from build123d import *

# Parameters (mm, degrees)
SKETCH1_R               = 4.75
BOSS_EXTRUDE1_DEPTH     = 9.5
SKETCH2_W               = 19
SKETCH2_H               = 9.5
CUT_EXTRUDE1_DEPTH      = 11
CUT_EXTRUDE1_DEPTH_BACK = 11
CHAMFER1_SIZE           = 8
CHAMFER1_SIZE2          = 1.895543273
CHAMFER2_SIZE           = 8
CHAMFER2_SIZE2          = 1.846945529
SKETCH5_R               = 1.5
CUT_EXTRUDE2_DEPTH      = 10.5000001
CUT_EXTRUDE2_DEPTH_BACK = 10.5000001


with BuildPart() as part:
    # Sketch1 → Boss-Extrude1 (new body, symmetric)
    with BuildSketch(Plane.XY):
        with BuildLine():
            Line((0, 10), (-22, 10))
            Line((-22, 10), (-22, 5))
            Line((-22, 5), (-9.9979998, 0.2))
            ThreePointArc((-9.9979998, 0.2), (-6.49865122, -7.600495531), (1.750767609, -9.845547866))
            Line((1.750767609, -9.845547866), (29, -5))
            Line((29, -5), (29, 0))
            Line((29, 0), (10, 0))
            ThreePointArc((10, 0), (7.071067812, 7.071067812), (0, 10))
        make_face()
        Circle(SKETCH1_R, mode=Mode.SUBTRACT)
    extrude(amount=BOSS_EXTRUDE1_DEPTH, both=True)

    # Sketch2 → Cut-Extrude1 (cut, two sides)
    with BuildSketch(Plane(origin=(0, 0, 0), x_dir=(1, 0, 0), z_dir=(0, 1, 0))) as cut_extrude1_sk:
        with Locations((-22, 0)):
            Rectangle(SKETCH2_W, SKETCH2_H)
        with Locations((29, 0)):
            Rectangle(SKETCH2_W, SKETCH2_H)
        with BuildLine():
            Line((-6, 5), (4, 5))
            ThreePointArc((4, 5), (9, 0), (4, -5))
            Line((4, -5), (-6, -5))
            ThreePointArc((-6, -5), (-11, 0), (-6, 5))
        make_face()
    extrude(amount=CUT_EXTRUDE1_DEPTH, mode=Mode.SUBTRACT)
    extrude(cut_extrude1_sk.sketch, amount=-CUT_EXTRUDE1_DEPTH_BACK, mode=Mode.SUBTRACT)

    # Chamfer1
    chamfer1_edges = [part.edges().sort_by_distance(p)[0] for p in [
        (-22, 7.5, 9.5),
        (29, -2.5, 9.5),
    ]]
    chamfer1_side = [part.faces().sort_by_distance(p)[0] for p in [
        (6.683704933, 6.683704933, 9.5),
    ]]
    chamfer(chamfer1_edges, length=CHAMFER1_SIZE, length2=CHAMFER1_SIZE2, reference=chamfer1_side[0])

    # Chamfer2
    chamfer2_edges = [part.edges().sort_by_distance(p)[0] for p in [
        (-22, 7.5, -9.5),
        (29, -2.5, -9.5),
    ]]
    chamfer2_side = [part.faces().sort_by_distance(p)[0] for p in [
        (6.683704933, 6.683704933, -9.5),
    ]]
    chamfer(chamfer2_edges, length=CHAMFER2_SIZE, length2=CHAMFER2_SIZE2, reference=chamfer2_side[0])

    # Sketch5 → Cut-Extrude2 (cut, two sides)
    with BuildSketch(Plane.XY) as cut_extrude2_sk:
        with Locations((-19.684598733, 7.5)):
            Circle(SKETCH5_R)
        with Locations((26.44619669, -2.5)):
            Circle(SKETCH5_R)
    extrude(amount=CUT_EXTRUDE2_DEPTH, mode=Mode.SUBTRACT)
    extrude(cut_extrude2_sk.sketch, amount=-CUT_EXTRUDE2_DEPTH_BACK, mode=Mode.SUBTRACT)


solid = part.part
Check sheet for the modelled part. Datum: model origin and axes. Units: mm. A direction names the side the tool comes from. Round coordinates to 2 decimals unless told otherwise and drop trailing zeros. Loops run counter-clockwise (first coordinate to the right, second up) from the corner with the lowest first, then second, coordinate; pieces in that order, holes last.
1. Gauge pin test, flat ends, axial feed: pin 1 Ø1 at (y, z) = (2.5, 3.5) entering from -X; pin 2 Ø8 at (y, z) = (-5.5, -2) entering from -X; pin 3 Ø5.5 at (x, y) = (26.5, -4.5) entering from +Z; pin 4 Ø2.5 at (x, y) = (-19.68, 7.5) entering from -Z. Record the tip position at first contact, or that the pin passes through.
2. Sectioned sample at D-D on y = 3.5. Record the boundary of the cut face in (x, z), and give its area (3 significant figures).
3. Sectioned sample at A-A on z = -0.5. Record the boundary of the cut face in (x, y).
4. Set-up check for faces 1 (the flat face through (-16, 7, 4.75)), 2 (the flat face through (18, 0, 0)), 3 (the flat face through (23, -3, 4.75)): record each of +Z, -Z, +X, -X, +Y, -Y from which the full face is reachable in a straight line by a thin tool's end or side.
5. Sectioned sample at C-C on x = 6. Record the boundary of the cut face in (y, z).
6. Mould release check, pull along Y, two halves, no side actions. Record for faces 4 (the flat face through (24.17, -3.26, -8.77)), 5 (the cylindrical face through (9.109, 4.126, 2.244)), 6 (the cylindrical face through (24.948, -2.434, 6.647)): released by +Y, released by -Y, zero draft, split by the parting line, or undercut.
7. Scan lines: probe 1 along Z at (x, y) = (-0.5, 8.5); probe 2 along X at (y, z) = (-2.5, 7.45); probe 3 along Z at (x, y) = (-13, 3). Record each from-to range of solid material in increasing order.
8. Sectioned sample at B-B on y = 7.5. Record the boundary of the cut face in (x, z), and give its area (3 significant figures).
Recorded:
1. pin 1: stops at x = -12.5
1. pin 2: stops at x = -9.86
1. pin 3: stops at z = 8.85
1. pin 4: passes through
2. outline: (-18.25, -8.52) - (-14, -9.5) - (-3.21, -9.5) - (-3.21, -5) - (-6, -5) arc R5 cw to (-6, 5) - (-3.21, 5) - (-3.21, 9.5) - (-14, 9.5) - (-18.25, 8.49) - (-18.25, 4.75) - (-12.5, 4.75) - (-12.5, -4.75) - (-18.25, -4.75) - close; (3.21, -9.5) - (9.37, -9.5) - (9.37, 9.5) - (3.21, 9.5) - (3.21, 5) - (4, 5) arc R5 cw to (4, -5) - (3.21, -5) - close
2. area: 230 mm2
3. outline: (-12.5, 1.2) - (-10.97, 0.59) - (-10.97, 10) - (-12.5, 10) - close; (8.97, -8.56) - (19.5, -6.69) - (19.5, 0) - (10, 0) arc R10 ccw to (8.97, 4.41) - close
4. face 1: -X, +Y, -Y
4. face 2: +Z, -Z, +X, +Y
4. face 3: +X, +Y, -Y
5. outline: (-9.09, -9.5) - (8, -9.5) - (8, -4.58) - (-9.09, -4.58) - close; (-9.09, 4.58) - (8, 4.58) - (8, 9.5) - (-9.09, 9.5) - close
6. face 4: zero draft
6. face 5: released by +Y
6. face 6: undercut
7. probe 1: z = -9.5 to -5, 5 to 9.5
7. probe 2: x = -9.68 to -4.04, 4.04 to 24.95, 27.95 to 29
7. probe 3: z = -9.5 to -4.75, 4.75 to 9.5
8. outline: (-22, -7.65) - (-21.18, -7.84) - (-21.18, -4.75) - (-22, -4.75) - close; (-22, 4.75) - (-21.18, 4.75) - (-21.18, 7.8) - (-22, 7.6) - close; (-18.18, -8.53) - (-14, -9.5) - (6.61, -9.5) - (6.61, -4.26) arc R5 cw to (4, -5) - (-6, -5) arc R5 cw to (-6, 5) - (4, 5) arc R5 cw to (6.61, 4.26) - (6.61, 9.5) - (-14, 9.5) - (-18.18, 8.51) - (-18.18, 4.75) - (-12.5, 4.75) - (-12.5, -4.75) - (-18.18, -4.75) - close
8. area: 254 mm2
